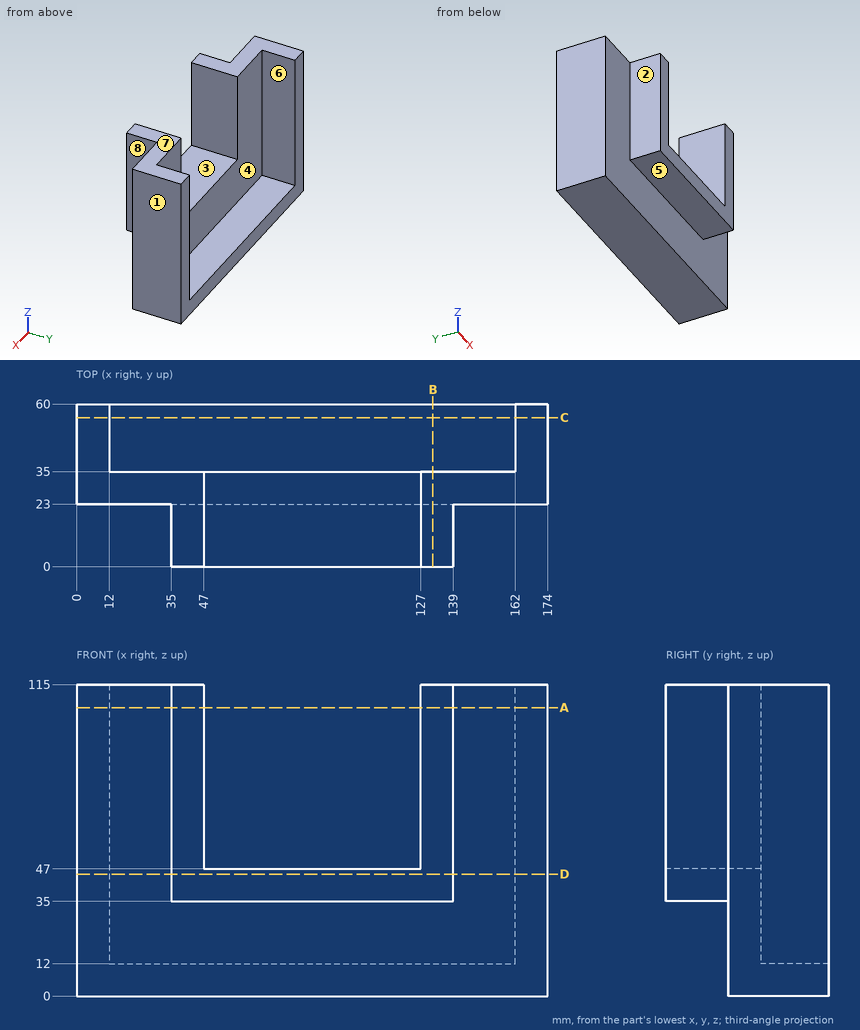
Geometry check sheet. Reference: drawing and pictorial views, mm from the part's lowest x, y, z. A direction names the side the tool comes from. Give positions to 0.01 mm unless a question says otherwise; leave off trailing zeros. Order: outer loops, then holes, each group sorted by start corner. A loop starts at its lowest first (then second) coordinate and runs counter-clockwise, first axis right, second up. Notation, with made-up numbers: M 70,14.25 L 91,14.25 A36 ccw 91,52.25 Z; hole C 54,-6.75 d11. An arc over 180 degrees is marked long. Answer as a JSON object with one key per item and string values. Group by question number.
1) Cross-section at A-A (z = 106.5). Enter the section's corners in (x, y), then the cut area to 3 significant figures.
2) Cross-section at B-B (x = 131.5). Enter the section's corners in (y, z).
3) Scan lines: line 1 along X through (y, z) = (57.5, 75); line 2 along X through (y, z) = (14.5, 79); line 3 along Z through (x, y) = (126.5, 22). Record each from-to range of solid material in increasing order. Write a range as [from, to].
4) Access from +Z, -Z, +X, -X, +Y, -Y to the whole of each face (thin tool, end or side, straight path). Record for the marked faces 1, 2, 3, 4 and 5.
5) Depth check by flat-ended pin: pin 1 Ø7.5 at (y, z) = (53, 58) entering from -X; pin 2 Ø5 at (x, z) = (152.5, 79.5) entering from +Y; pin 3 Ø18.5 at (x, y) = (103, 12) entering from -Z; pin 4 Ø1 at (x, y) = (91, 48) entering from +Z. Enter the tip coordinate at first touch or a pass-through.
6) Cross-section at C-C (y = 55). Enter the section's corners in (x, z), then the cut area to 3 significant figures.
7) Cross-section at D-D (z = 45). Enter the section's corners in (x, y).
8) Mould release check, pull along X, two halves, no side actions. Record for the marked faces 6, 7 and 8: released by +X, released by -X, zero draft, split by the parting line, or undercut.
Result sheet:
{
 "1": {"outline": "M 0,23 L 35,23 L 35,0 L 47,0 L 47,35 L 12,35 L 12,60 L 0,60 Z; M 127,0 L 139,0 L 139,23 L 174,23 L 174,60 L 162,60 L 162,35 L 127,35 Z", "area": "2,280 mm2"},
 "2": {"outline": "M 0,35 L 23,35 L 23,0 L 60,0 L 60,12 L 35,12 L 35,115 L 0,115 Z"},
 "3": {"line 1": "x = [0, 12], [162, 174]", "line 2": "x = [35, 47], [127, 139]", "line 3": "z = [35, 47]"},
 "4": {"face 1": "+Z, -Z, +X, +Y, -Y", "face 2": "+Z, -Z, -X, -Y", "face 3": "+Z, +Y, -Y", "face 4": "+Z, +Y", "face 5": "-Z, +X, -X, -Y"},
 "5": {"pin 1": "stops at x = 0", "pin 2": "stops at y = 35", "pin 3": "stops at z = 35", "pin 4": "stops at z = 12"},
 "6": {"outline": "M 0,0 L 174,0 L 174,115 L 162,115 L 162,12 L 12,12 L 12,115 L 0,115 Z", "area": "4,560 mm2"},
 "7": {"outline": "M 0,23 L 35,23 L 35,0 L 139,0 L 139,23 L 174,23 L 174,60 L 162,60 L 162,35 L 12,35 L 12,60 L 0,60 Z"},
 "8": {"face 6": "undercut", "face 7": "zero draft", "face 8": "released by +X"}
}
